```python
from build123d import *

# Parameters (mm, degrees)
F0_W      = 111.125
F0_H      = 9.525
F1_DEPTH  = 53.975
F3_DEPTH  = 9.526
F4_W      = 9.525
F4_H      = 44.45
F5_DEPTH  = 50.8
F7_DEPTH  = 63.501
F9_DEPTH  = 9.526
F10_R     = 6.35
F11_DEPTH = 9.526
F13_DEPTH = 9.526


with BuildPart() as f1:
    # F0 (on Front) → F1 (new body)
    with BuildSketch(Plane.XZ):
        with Locations((16.7216053668, -25.4447730258)):
            Rectangle(F0_W, F0_H)
    extrude(amount=-F1_DEPTH)

    # F2 (on face) → F3 (cut, through all)
    with BuildSketch(Plane.XY.offset(-20.6822730258)):
        Polygon((15.1341053668, 0), (-38.8408946332, 34.925), (-38.8408946332, 0), align=None)
    extrude(amount=-F3_DEPTH, mode=Mode.SUBTRACT)

    # F4 (on face) → F5 (join)
    with BuildSketch(Plane.XY.offset(-20.6822730258)):
        with Locations((19.8966053668, 22.225)):
            Rectangle(F4_W, F4_H)
        Polygon((72.2841053668, 44.45), (72.2841053668, 53.975), (-38.8408946332, 53.975), (-38.8408946332, 44.45), (15.1341053668, 44.45), (24.6591053668, 44.45), align=None)
    extrude(amount=F5_DEPTH)

    # F6 (on face) → F7 (cut, through all)
    with BuildSketch(Plane.YZ.offset(24.6591053668)):
        Polygon((0, 30.1177269742), (0, -20.6822730258), (44.45, 30.1177269742), align=None)
    extrude(amount=-F7_DEPTH, mode=Mode.SUBTRACT)

    # F8 (on face) → F9 (cut, through all)
    with BuildSketch(Plane.XZ.offset(-44.45)):
        Polygon((72.2841053668, 30.1177269742), (24.6591053668, 30.1177269742), (72.2841053668, -20.6822730258), align=None)
    extrude(amount=-F9_DEPTH, mode=Mode.SUBTRACT)

    # F10 (on face) → F11 (cut, through all)
    with BuildSketch(Plane.XY.offset(-20.6822730258)):
        with Locations((37.3591053668, 22.225)):
            Circle(F10_R)
        with Locations((59.5841053668, 22.225)):
            Circle(F10_R)
    extrude(amount=-F11_DEPTH, mode=Mode.SUBTRACT)

    # F12 (on face) → F13 (cut, through all)
    with BuildSketch(Plane.XZ.offset(-44.45)):
        Polygon((-22.9658946332, 14.2427269742), (-28.5221446332, 14.2427269742), (-28.5221446332, -4.8072730258), (-17.4096446332, -4.8072730258), (-17.4096446332, 14.2427269742), align=None)
        with BuildLine():
            ThreePointArc((-17.4096446332, 14.2427269742), (-22.9658946332, 19.7989769742), (-28.5221446332, 14.2427269742))
            Line((-28.5221446332, 14.2427269742), (-22.9658946332, 14.2427269742))
            Line((-22.9658946332, 14.2427269742), (-17.4096446332, 14.2427269742))
        make_face()
        with BuildLine():
            Line((4.8153553668, -4.8072730258), (-6.2971446332, -4.8072730258))
            ThreePointArc((-6.2971446332, -4.8072730258), (-0.7408946332, -10.3635230258), (4.8153553668, -4.8072730258))
        make_face()
        Polygon((-0.7408946332, 14.2427269742), (-6.2971446332, 14.2427269742), (-6.2971446332, -4.8072730258), (4.8153553668, -4.8072730258), (4.8153553668, 14.2427269742), align=None)
        with BuildLine():
            ThreePointArc((4.8153553668, 14.2427269742), (-0.7408946332, 19.7989769742), (-6.2971446332, 14.2427269742))
            Line((-6.2971446332, 14.2427269742), (-0.7408946332, 14.2427269742))
            Line((-0.7408946332, 14.2427269742), (4.8153553668, 14.2427269742))
        make_face()
        with BuildLine():
            Line((-17.4096446332, -4.8072730258), (-28.5221446332, -4.8072730258))
            ThreePointArc((-28.5221446332, -4.8072730258), (-22.9658946332, -10.3635230258), (-17.4096446332, -4.8072730258))
        make_face()
    extrude(amount=-F13_DEPTH, mode=Mode.SUBTRACT)


solid = f1.part
```
Model file for the job. Use its own axes, mm. A direction names the side the tool comes from. Coordinates: 2 decimals unless noted, no trailing zeros. Order: outer loops, then holes, each group sorted by start corner. A loop starts at its lowest first (then second) coordinate and runs counter-clockwise, first axis right, second up. Notation, with made-up numbers: (8.25, 76.25) - (37.25, 76.25) arc R27 ccw to (37.25, 92.25) - close; hole circle Ø1 at (68.25, -31.5). An arc over 180 degrees is marked (long way). Return JSON: item names as keys, results as strings. Group by question number.
1) Saw through at C-C, the plane x = -3.5. Write the cut outline in (y, z) (3 decimals), plus the area to 3 significant figures.
2) Tool access for faces 4 (the flat face through (72.284, 27, -26)), 5 (the flat face through (-6, 27, -20.682)), 6 (the flat face through (-38.841, 49, 0)), 7 (the flat face through (48, 22, -20.682)), 8 (the flat face through (-6.297, 49, 5)): list every direction of +Z, -Z, +X, -X, +Y, -Y with a clear straight run to the whole face (end or side of a thin tool).
3) Saw through at A-A, the plane y = 46. Write the cut outline in (x, z).
4) Flat gauge pins, fed straight in: P1, Ø7.5, axis at y = 47, z = 8.5, coming from the +X side; P2, Ø7.5, axis at y = 50.5, z = 7.5, coming from the +X side; P3, Ø5, axis at x = 0, y = 39, coming from the +Z side. Where does each tip first touch, or does it go through?
5) Saw through at B-B, the plane z = 18. Write the cut outline in (x, y) (3 decimals).
6) Mould opens along Y. For faces 1 (the flat face through (15.134, 32, -7)), 2 (the cylindrical face through (62.51, 16.59, -25.38)), 3 (the flat face through (-12, 44.45, 4)) say: released by +Y, released by -Y, zero draft, split by the parting line, or undercut.
7) Saw through at D-D, the plane z = -16.5. Write the cut outline in (x, y) (3 decimals).
8) Probe line 1 (X direction, y = 47.5, z = -6.5); line 2 (Z direction, x = 32, y = 26); line 3 (X direction, y = 24, z = -10). List the from-to ranges inside material, lowest first. Write a range as from..to.
Values found:
{
 "1": {"outline": "(12.057, -30.207) - (53.975, -30.207) - (53.975, -9.63) - (44.45, -9.63) - (44.45, -20.682) - (12.057, -20.682) - close; (44.45, 19.066) - (53.975, 19.066) - (53.975, 30.118) - (44.45, 30.118) - close", "area": "610 mm²"},
 "2": {"face 4": "+Z, -Z, +X, +Y, -Y", "face 5": "+Z, -X, -Y", "face 6": "+Z, -Z, -X, +Y, -Y", "face 7": "+Z, +X, -Y", "face 8": "+Y, -Y"},
 "3": {"outline": "(-38.84, -30.21) - (72.28, -30.21) - (72.28, -20.68) - (24.66, 30.12) - (-38.84, 30.12) - close; hole (-28.52, -4.81) arc R5.56 ccw to (-17.41, -4.81) - (-17.41, 14.24) arc R5.56 ccw to (-28.52, 14.24) - close; hole (-6.3, -4.81) arc R5.56 ccw to (4.82, -4.81) - (4.82, 14.24) arc R5.56 ccw to (-6.3, 14.24) - close"},
 "4": {"P1": "stops at x = 48.44", "P2": "stops at x = 49.38", "P3": "stops at z = -20.68"},
 "5": {"outline": "(-38.841, 44.45) - (-27.059, 44.45) - (-27.059, 53.975) - (-38.841, 53.975) - close; (-18.873, 44.45) - (-4.834, 44.45) - (-4.834, 53.975) - (-18.873, 53.975) - close; (3.352, 44.45) - (15.134, 44.45) - (15.134, 33.847) - (24.659, 33.847) - (24.659, 44.45) - (36.019, 44.45) - (36.019, 53.975) - (3.352, 53.975) - close"},
 "6": {"face 1": "zero draft", "face 2": "undercut", "face 3": "released by -Y"},
 "7": {"outline": "(-38.841, 44.45) - (15.134, 44.45) - (15.134, 3.659) - (24.659, 3.659) - (24.659, 44.45) - (68.363, 44.45) - (68.363, 53.975) - (-38.841, 53.975) - close"},
 "8": {"line 1": "x = -38.84..-28.26, -17.67..-6.03, 4.55..58.99", "line 2": "z = -30.21..-20.68", "line 3": "x = 15.13..24.66"}
}
